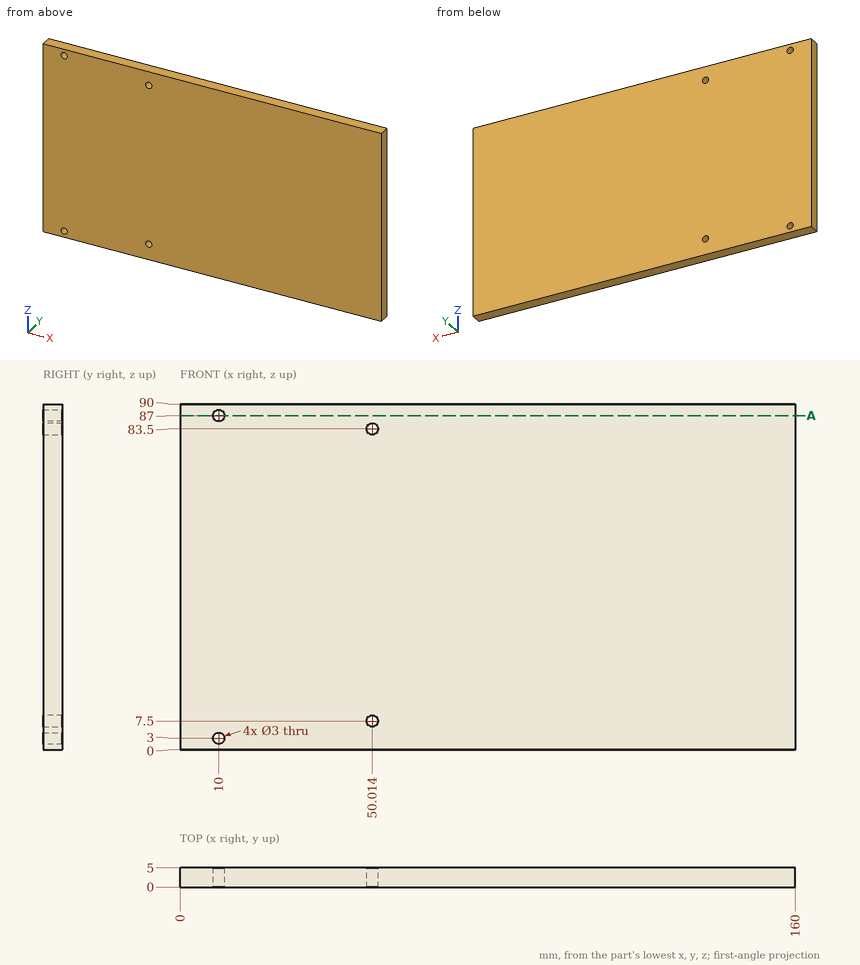
Study the drawing (mm; zero at the part's minimum x, y, z) and answer. Coordinates: 2 decimals unless noted, no trailing zeros. Loops run counter-clockwise (first coordinate to the right, second up) from the corner with the lowest first, then second, coordinate; pieces in that order, holes last. Notation, with made-up numbers: (-24, 88.25) -> (24, 88.25) arc R29 cw to (24, 121.25) -> close; hole circle Ø3 at (73.5, 32). An arc over 180 degrees is marked (long way). Answer in a Markdown table with one row per item. Add a question column.
1. The part is cut by section A-A, the plane z = 87. Write down the section's boundary in (x, y), then the cut area to 3 significant figures.
2. Flat-ended cylindrical pins translate along their axes: P1, Ø6, axis at x = 48, z = 60.5, coming from the -Y side; P2, Ø2.5, axis at x = 10, z = 3, coming from the +Y side. Find the tip coordinate at first contact, or state that the pin passes through.
3. Consider line 1 (X direction, y = 3.3, z = 7.5); line 2 (X direction, y = 2.75, z = 3). Determine where each line is inside the solid, lowest interval first. Write a range as [from, to].
Answer below:
| question | item | result |
|---|---|---|
| 1 | outline | (0, 0) -> (8.5, 0) -> (8.5, 5) -> (0, 5) -> close; (11.5, 0) -> (160, 0) -> (160, 5) -> (11.5, 5) -> close |
| 1 | area | 785 mm2 |
| 2 | P1 | y = 0 |
| 2 | P2 | through |
| 3 | line 1 | [0, 48.51], [51.51, 160] |
| 3 | line 2 | [0, 8.5], [11.5, 160] |
